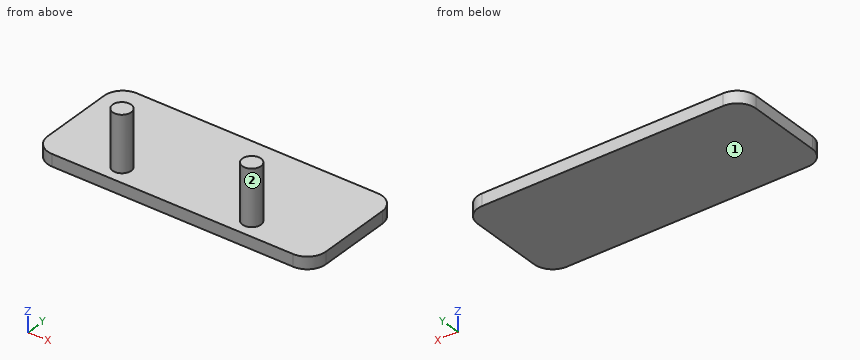
```python
from build123d import *

# Parameters (mm, degrees)
F1_DEPTH = 4.1275
F2_R     = 3.175
F3_DEPTH = 19.05


with BuildPart() as f1:
    # F0 (on Top) → F1 (new body)
    with BuildSketch(Plane.XY):
        with BuildLine():
            ThreePointArc((0, 6.35), (1.859872, 1.859872), (6.35, 0))
            Line((6.35, 0), (88.9, 0))
            ThreePointArc((88.9, 0), (93.390128, 1.859872), (95.25, 6.35))
            Line((95.25, 6.35), (95.25, 31.75))
            ThreePointArc((95.25, 31.75), (93.390128, 36.240128), (88.9, 38.1))
            Line((88.9, 38.1), (6.35, 38.1))
            ThreePointArc((6.35, 38.1), (1.859872, 36.240128), (0, 31.75))
            Line((0, 31.75), (0, 6.35))
        make_face()
    extrude(amount=F1_DEPTH)

    # F2 (on face) → F3 (join)
    with BuildSketch(Plane.XY.offset(4.1275)):
        with Locations((25.4, 6.35)):
            Circle(F2_R)
        with Locations((69.85, 6.35)):
            Circle(F2_R)
    extrude(amount=F3_DEPTH)


solid = f1.part
```
The listing builds one solid part. Answer for the finished solid, in the listing's coordinates (mm). Face numbers are marked on the shaded views. Give positions to 0.01 mm unless a question says otherwise; leave off trailing zeros. Order: outer loops, then holes, each group sorted by start corner. A loop starts at its lowest first (then second) coordinate and runs counter-clockwise, first axis right, second up. Notation, with made-up numbers: (-21.75, -11) - (2.25, -11) arc R8 cw to (2.25, -5) - close; hole circle Ø3 at (-4.75, -10.75). An arc over 180 degrees is marked (long way). Answer in a Markdown table with one row per item. Add a question column.
Q1. The part is cut by section B-B (z = 8.5). Determine the outline of the cut face in (x, y) (3 decimals), then the cut area to 3 significant figures.
Q2. For a pull along X with two mould halves and no side action, classify the marked faces 1 and 2 as released by +X, released by -X, zero draft, split by the parting line, or undercut.
Q3. The part is cut by section A-A (x = 25.4). Determine the outline of the cut face in (y, z) (1 decimal).
Q4. The part is cut by section C-C (y = 30). Determine the outline of the cut face in (x, z).
Q5. Find the intervals of material crossed by line 1 along Z through (x, y) = (18, 19.5); line 2 along X through (y, z) = (6.5, 10.25); line 3 along X through (y, z) = (7, 16.75), in increasing order. Write a range as [from, to].
Q6. The part is cut by section D-D (x = 47.5). Determine the outline of the cut face in (y, z), then the cut area to 3 significant figures.
Q7. Given P1, Ø2, axis at x = 24.5, y = 16, coming from the +Z side; P2, Ø4, axis at x = 69, z = 7.5, coming from the -Y side (3 decimals); P3, Ø5, axis at y = 5, z = 17.5, coming from the +X side (3 decimals), each flat-ended and moving along its own axis, determine where each tip first touches the part or whether it passes through.
Determined:
| question | item | result |
|---|---|---|
| 1 | outline | circle Ø6.35 at (25.4, 6.35); circle Ø6.35 at (69.85, 6.35) |
| 1 | area | 63.3 mm² |
| 2 | face 1 | zero draft |
| 2 | face 2 | undercut |
| 3 | outline | (0, 0) - (38.1, 0) - (38.1, 4.1) - (9.5, 4.1) - (9.5, 23.2) - (3.2, 23.2) - (3.2, 4.1) - (0, 4.1) - close |
| 4 | outline | (0, 0) - (95.25, 0) - (95.25, 4.13) - (0, 4.13) - close |
| 5 | line 1 | z = [0, 4.13] |
| 5 | line 2 | x = [22.23, 28.57], [66.68, 73.02] |
| 5 | line 3 | x = [22.29, 28.51], [66.74, 72.96] |
| 6 | outline | (0, 0) - (38.1, 0) - (38.1, 4.13) - (0, 4.13) - close |
| 6 | area | 157 mm² |
| 7 | P1 | stops at z = 4.13 |
| 7 | P2 | stops at y = 3.175 |
| 7 | P3 | stops at x = 73.025 |
